Model file for the job. Use its own axes, mm. A direction names the side the tool comes from. Round coordinates to 2 decimals unless told otherwise and drop trailing zeros. Loops run counter-clockwise (first coordinate to the right, second up) from the corner with the lowest first, then second, coordinate; pieces in that order, holes last. Notation, with made-up numbers: M 86.25,56.5 L 97.25,56.5 A22 cw 97.25,75.5 Z; hole C 13,81.5 d5. An arc over 180 degrees is marked long. Use a Markdown table: item, result. Add a question column.
Q1. Mould opens along Y. For faces 1 (the face through (22.026, 8.852, -1.972)), 2 (the face through (10, 15, -11)), 3 (the face through (10, 7, 0)) say: +Y half, -Y half, draft (parallel to the pull), parting line (faces both ways), or undercut.
Q2. Cut at C-C (y = 10.75). Give the cut face in (x, z).
Q3. Tool access for faces 4 (the face through (2.5, 7, -13)), 5 (the face through (22.1, 5.7, -4)), 6 (the face through (29.5, 8, -2)): list every direction of +Z, -Z, +X, -X, +Y, -Y with a clear straight run to the whole face (end or side of a thin tool).
Q4. Pin check, flat tips, straight feed: pin 1 (1.5 mm diameter, centred on y = 5, z = -16.5, fed in from -X); pin 2 (4.5 mm diameter, centred on x = -3.5, y = 7.5, fed in from -Z); pin 3 (4.5 mm diameter, centred on y = 9, z = -11.5, fed in from +X). Stop position of each tip, or through.
Q5. Probe line 1 (Y direction, x = -3.5, z = -1.1); line 2 (X direction, y = 13, z = -25.75); line 3 (X direction, y = 1, z = -15). List the from-to ranges inside material, lowest first. Write a range as from..to.
Q6. Cut at A-A (y = 7.5). Give the cut face in (x, z), plus the area to 3 significant figures.
Q7. Cut at B-B (x = 10). Give the cut face in (y, z), plus the area to 4 significant figures.
Q8. Cut at D-D (z = -17.5). Give the cut face in (x, y).
from build123d import *

# Parameters (mm, degrees)
BOSS_EXTRU_1_DEPTH      = 15
BOSS_EXTRU_2_DEPTH      = 12
BOSS_EXTRU_2_DEPTH_BACK = 27
ESQUISSE2_W             = 4
ESQUISSE2_H             = 15
ESQUISSE3_R             = 2
ENL_V_MAT_EXTRU_1_DEPTH = 12


with BuildPart() as part:
    # Esquisse1 → Boss.-Extru.1 (new body)
    with BuildSketch(Plane(origin=(0, 0, 0), x_dir=(1, 0, 0), z_dir=(0, 1, 0))):
        with BuildLine():
            ThreePointArc((17.5, 22), (10, 29.5), (2.5, 22))
            Line((2.5, 22), (5, 22))
            ThreePointArc((5, 22), (10, 27), (15, 22))
            Line((15, 22), (17.5, 22))
        make_face()
        with BuildLine():
            Line((5, 22), (2.5, 22))
            ThreePointArc((2.5, 22), (10, 14.5), (17.5, 22))
            Line((17.5, 22), (15, 22))
            ThreePointArc((15, 22), (10, 17), (5, 22))
        make_face()
        with BuildLine():
            Line((2.5, 22), (2.5, 0))
            Line((2.5, 0), (17.5, 0))
            Line((17.5, 0), (17.5, 22))
            ThreePointArc((17.5, 22), (10, 14.5), (2.5, 22))
        make_face()
    extrude(amount=BOSS_EXTRU_1_DEPTH)

    # Esquisse2 → Boss.-Extru.2 (add, two sides: drawn at the far end of the back side and taken through both)
    with BuildSketch(Plane(origin=(17.5, 0, 0), x_dir=(0, 0, -1), z_dir=(1, 0, 0)).offset(-BOSS_EXTRU_2_DEPTH_BACK)):
        with Locations((2, 7.5)):
            Rectangle(ESQUISSE2_W, ESQUISSE2_H)
    extrude(amount=BOSS_EXTRU_2_DEPTH + BOSS_EXTRU_2_DEPTH_BACK)

    # Esquisse3 → Enlèv. mat.-Extru.1 (cut)
    with BuildSketch(Plane.XY):
        with Locations((-3.5, 7.5)):
            Circle(ESQUISSE3_R)
        with Locations((23.5, 7.5)):
            Circle(ESQUISSE3_R)
    extrude(amount=-ENL_V_MAT_EXTRU_1_DEPTH, mode=Mode.SUBTRACT)


solid = part.part
Checked values:
| question | item | result |
|---|---|---|
| 1 | face 1 | undercut |
| 1 | face 2 | +Y half |
| 1 | face 3 | draft |
| 2 | outline | M -9.5,-4 L 2.5,-4 L 2.5,-22 A7.5 ccw 17.5,-22 L 17.5,-4 L 29.5,-4 L 29.5,0 L -9.5,0 Z; hole C 10,-22 d10 |
| 3 | face 4 | -Z, -X, +Y, -Y |
| 3 | face 5 | -Z, +X, +Y, -Y |
| 3 | face 6 | +Z, -Z, +X, +Y, -Y |
| 4 | pin 1 | stops at x = 2.5 |
| 4 | pin 2 | stops at z = -4 |
| 4 | pin 3 | stops at x = 17.5 |
| 5 | line 1 | y = 0..5.5, 9.5..15 |
| 5 | line 2 | x = 3.5..6.69, 13.31..16.5 |
| 5 | line 3 | x = 2.5..17.5 |
| 6 | outline | M -9.5,-4 L -5.5,-4 L -5.5,0 L -9.5,0 Z; M -1.5,-4 L 2.5,-4 L 2.5,-22 A7.5 ccw 17.5,-22 L 17.5,-4 L 21.5,-4 L 21.5,0 L -1.5,0 Z; M 25.5,-4 L 29.5,-4 L 29.5,0 L 25.5,0 Z; hole C 10,-22 d10 |
| 6 | area | 404 mm^2 |
| 7 | outline | M 0,-29.5 L 15,-29.5 L 15,-27 L 0,-27 Z; M 0,-17 L 15,-17 L 15,0 L 0,0 Z |
| 7 | area | 292.5 mm^2 |
| 8 | outline | M 2.5,0 L 7.82,0 L 7.82,15 L 2.5,15 Z; M 12.18,0 L 17.5,0 L 17.5,15 L 12.18,15 Z |
